from build123d import *

# Parameters (mm, degrees)
BOSS_EXTRUDE1_DEPTH = 1.5875
BOSS_EXTRUDE2_DEPTH = 1.5875


with BuildPart() as part:
    # Sketch1 → Boss-Extrude1 (new body)
    with BuildSketch(Plane.XY):
        with BuildLine():
            Line((40.005, -76.2), (40.005, -25.840677236))
            ThreePointArc((40.005, -25.840677236), (45.68029526, -13.470384182), (47.625, 0))
            Line((47.625, 0), (47.625, 12.7))
            Line((47.625, 12.7), (186.055, 12.7))
            Line((186.055, 12.7), (186.055, 0))
            Line((186.055, 0), (186.055, -76.2))
            ThreePointArc((186.055, -76.2), (113.03, -149.225), (40.005, -76.2))
        make_face()
    extrude(amount=BOSS_EXTRUDE1_DEPTH)

    # Sketch2 → Boss-Extrude2 (add)
    with BuildSketch(Plane.XY):
        with BuildLine():
            Line((186.055, -76.2), (186.055, 0))
            Line((186.055, 0), (186.055, 12.7))
            Line((186.055, 12.7), (198.755, 12.7))
            Line((198.755, 12.7), (198.755, -76.2))
            ThreePointArc((198.755, -76.2), (113.03, -161.925), (27.305, -76.2))
            Line((27.305, -76.2), (27.305, -39.020220399))
            ThreePointArc((27.305, -39.020220399), (34.294082791, -33.046278315), (40.005, -25.840677236))
            Line((40.005, -25.840677236), (40.005, -76.2))
            ThreePointArc((40.005, -76.2), (113.03, -149.225), (186.055, -76.2))
        make_face()
    extrude(amount=BOSS_EXTRUDE2_DEPTH)


solid = part.part
Work out the finished part from the listing and answer in its coordinate system (mm). Coordinates: 2 decimals unless noted, no trailing zeros. Order: outer loops, then holes, each group sorted by start corner. A loop starts at its lowest first (then second) coordinate and runs counter-clockwise, first axis right, second up. Notation, with made-up numbers: (9, 8) - (39, 8) arc R24 ccw to (39, 22) - close; hole circle Ø4 at (21.5, 86). An arc over 180 degrees is marked (long way). Put each result on its own line as item: value. Start each with the question number.
1) Find section B-B (y = -20). Give the vertices of the cut face in (x, z) (1 decimal), plus the area to 3 significant figures.
2) Find section A-A (z = 0.25). Give the vertices of the cut face in (x, y) (3 decimals), plus the area to 3 significant figures.
3) Find the intervals of material crossed by line 1 (Y direction, x = 38.5, z = 0.8); line 2 (X direction, y = -120.5, z = 0.55); line 3 (X direction, y = -80, z = 1.05), in increasing order. Write a range as from..to.
4) Find section C-C (x = 153). Give the vertices of the cut face in (y, z), plus the area to 3 significant figures.
Results list:
1. outline: (43.2, 0) - (198.8, 0) - (198.8, 1.6) - (43.2, 1.6) - close
1. area: 247 mm^2
2. outline: (27.305, -76.2) arc R85.725 ccw to (198.755, -76.2) - (198.755, 12.7) - (47.625, 12.7) - (47.625, 0) arc R47.625 cw to (27.305, -39.02) - close
2. area: 26,000 mm^2
3. line 1: y = -118.56..-28.03
3. line 2: x = 39.64..186.42
3. line 3: x = 27.39..198.67
4. outline: (-152.04, 0) - (12.7, 0) - (12.7, 1.59) - (-152.04, 1.59) - close
4. area: 262 mm^2
